Autodesk Inventor part; units mm, degrees
ref_plane "YZ Plane" through (0, 0, 0) normal (1, 0, 0) x (0, 1, 0)
ref_plane "XZ Plane" through (0, 0, 0) normal (0, 1, 0) x (-1, 0, 0)
ref_plane "XY Plane" through (0, 0, 0) normal (0, 0, 1) x (1, 0, 0)
sketch "Sketch1" plane through (0, 0, 0) normal (0, 0, 1) x (1, 0, 0)
  line L0 (0, 0) -> (1219.2, 0)
  line L1 (1219.2, 0) -> (1219.2, 279.4)
  line L2 (0, 279.4) -> (0, 0)
  line L3 (381, 50.8) -> (0, 279.4)
  line L4 (838.2, 50.8) -> (1219.2, 279.4)
  line L5 (330.2, 152.0857) -> (330.5143, 152.4)
  line L6 (787.7143, 152.4) -> (787.4, 152.4)
  line L7 (127, 152.4) -> (126.6857, 152.4)
  line L8 (381, 50.8) -> (609.6, 165.1)
  line L9 (838.2, 50.8) -> (609.6, 165.1)
  dimension "d37" = 165.1
  dimension "d39" = 457.2
  dimension "d40" = 1219.2
  dimension "d41" = 381
  dimension "d43" = 279.4
  dimension "d44" = 279.4
  dimension "d45" = 50.8
  dimension "d46" = 50.8
  dimension "d47" = 228.6
extrude "Extrusion3" add sketch "Sketch1" against normal blind 1219.2
sketch "Sketch3" plane through (609.6, 165.1, 0) normal (-0.4472, 0.8944, 0) x (0.8944, 0.4472, 0)
  line L0 (-179.3826, 609.6) -> (0, 609.6)
  line L1 (0, 0) -> (0, 1219.2)
  line L2 (-255.5826, 1219.2) -> (0, 1219.2)
  line L3 (-179.3826, 1219.2) -> (-179.3826, 0)
  line L4 (-255.5826, 0) -> (-255.5826, 1219.2)
  point P0 (-619.0778, 0)
  dimension "d52" = 76.2
  dimension "d53" = 609.6
sketch "Sketch4" plane through (838.2, 50.8, 0) normal (0.4472, 0.8944, 0) x (0.8944, -0.4472, 0)
  line L0 (0, 1219.2) -> (238.5437, 1219.2)
  line L1 (-76.2, 609.6) -> (-255.5826, 609.6)
  line L2 (-255.5826, 0) -> (-255.5826, 1219.2)
  line L3 (0, 0) -> (-255.5826, 0)
  line L4 (-76.2, 0) -> (-76.2, 1219.2)
  line L5 (-255.5826, 1219.2) -> (0, 1219.2)
  line L6 (0, 0) -> (0, 1219.2)
  point P0 (-726.9904, 0)
  dimension "d54" = 76.2
sketch "Sketch5" plane through (1219.2, 279.4, 0) normal (-0.5145, 0.8575, 0) x (0.8575, 0.5145, 0)
  line L0 (0, 0) -> (0, 1219.2)
  line L1 (0, 609.6) -> (-444.3185, 609.6)
  line L2 (-444.3185, 0) -> (-444.3185, 1219.2)
  point P0 (-1189.2055, 0)
sketch "Sketch6" plane through (381, 50.8, 0) normal (0.5145, 0.8575, 0) x (0.8575, -0.5145, 0)
  line L0 (-444.3185, 0) -> (-444.3185, 1219.2)
  line L1 (-444.3185, 609.6) -> (0, 609.6)
  line L2 (0, 0) -> (0, 1219.2)
  point P0 (-300.5684, 0)
split_face "Split1"
split_face "Split2"
split_face "Split3"
split_face "Split4"
split_face "Split5"
split_face "Split6"
properties part number "Drone Charging Base" material "Aluminum 6061"
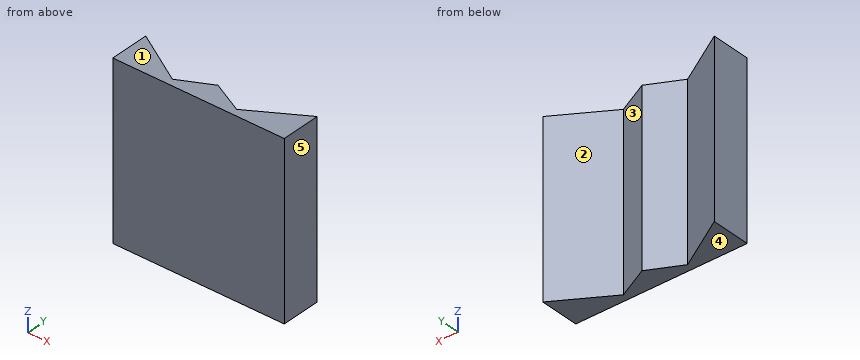
CAD build for the part. Positions are in the model's coordinates, mm. Face numbers are marked on the shaded views. A direction names the side the tool comes from. Give positions to 0.01 mm unless a question says otherwise; leave off trailing zeros. Order: outer loops, then holes, each group sorted by start corner. A loop starts at its lowest first (then second) coordinate and runs counter-clockwise, first axis right, second up.
(1) Mould opens along X. For the marked faces 3, 4 and 5 say: released by +X, released by -X, zero draft, split by the parting line, or undercut.
(2) Saw through at A-A, the plane y = 246. Give the cut face in (x, z), then the cut area to 3 significant figures.
(3) Saw through at B-B, the plane z = -115. Give the cut face in (x, y).
(4) Saw through at D-D, the plane x = 1070. Give the cut face in (y, z).
(5) Tool access for the marked faces 1 and 2: list every direction of +Z, -Z, +X, -X, +Y, -Y with a clear straight run to the whole face (end or side of a thin tool).
(6) Saw through at C-C, the plane y = 93.5. Give the cut face in (x, z), then the cut area to 3 significant figures.
(7) Drill centre lines: L1, parallel to X at y = 107.5, z = -494.5; L2, parallel to X at y = 104, z = -466; L3, parallel to X at y = 185, z = -1068.5. Where is each one in solid material? Low to high.
(8) Flat gauge pin, fed straight in: pin 1 (6 mm diameter, centred on x = 487.5, z = -780.5, fed in from +Y). Where does the tip first touch, or does it go through?
Results found:
1. face 3: undercut
1. face 4: zero draft
1. face 5: released by +X
2. outline: (0, -1219.2) - (55.67, -1219.2) - (55.67, 0) - (0, 0) - close; (1163.53, -1219.2) - (1219.2, -1219.2) - (1219.2, 0) - (1163.53, 0) - close
2. area: 136,000 mm2
3. outline: (0, 0) - (1219.2, 0) - (1219.2, 279.4) - (838.2, 50.8) - (609.6, 165.1) - (381, 50.8) - (0, 279.4) - close
4. outline: (0, -1219.2) - (189.88, -1219.2) - (189.88, 0) - (0, 0) - close
5. face 1: +Z, +X, -X, +Y, -Y
5. face 2: +Z, -Z, +Y
6. outline: (0, -1219.2) - (309.83, -1219.2) - (309.83, 0) - (0, 0) - close; (466.4, -1219.2) - (752.8, -1219.2) - (752.8, 0) - (466.4, 0) - close; (909.37, -1219.2) - (1219.2, -1219.2) - (1219.2, 0) - (909.37, 0) - close
6. area: 1,100,000 mm2
7. L1: x = 0 to 286.5, 494.4 to 724.8, 932.7 to 1219.2
7. L2: x = 0 to 292.33, 487.4 to 731.8, 926.87 to 1219.2
7. L3: x = 0 to 157.33, 1061.87 to 1219.2
8. pin 1: stops at y = 105.55
